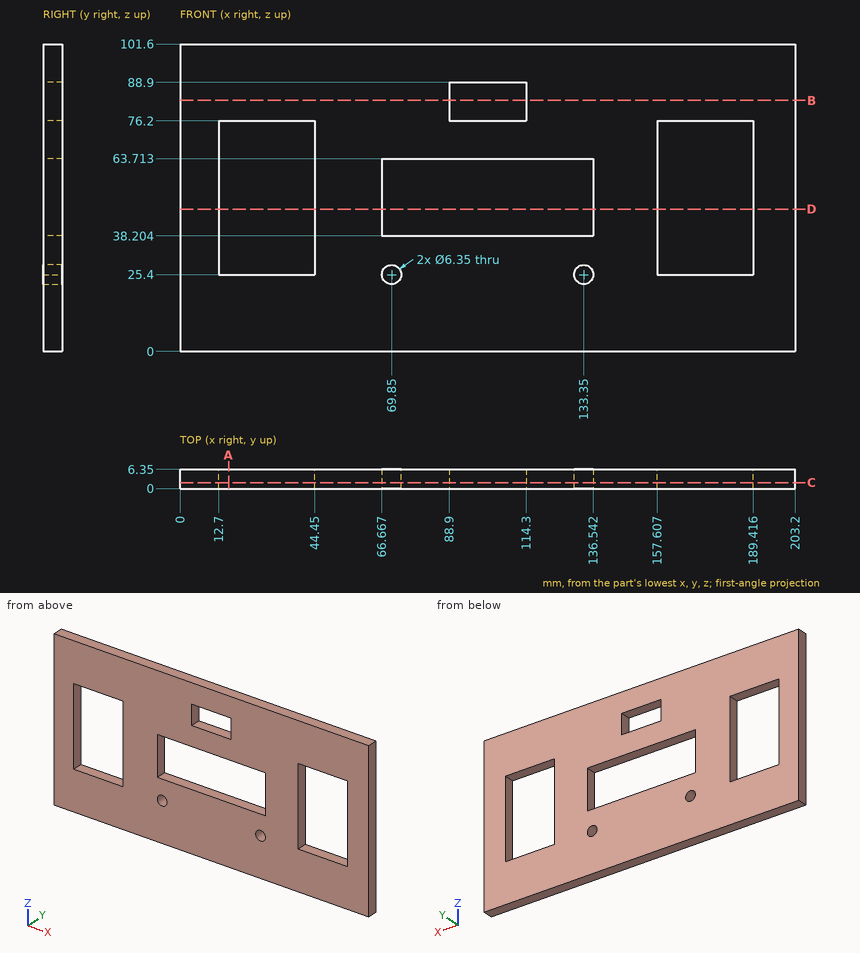
Job drawing, mm, ordinate dimensions from the low corner. One solid piece. Coordinates: 2 decimals unless noted, no trailing zeros. Order: outer loops, then holes, each group sorted by start corner. A loop starts at its lowest first (then second) coordinate and runs counter-clockwise, first axis right, second up. Notation, with made-up numbers: (60, 78.5) -> (97, 78.5) arc R25 cw to (97, 107.5) -> close; hole circle Ø10 at (43.5, -13). An arc over 180 degrees is marked (long way). Put each result on its own line as item: value. Start each with the question number.
(1) Band-saw the part on A-A (x = 16). Give the cut face in (y, z).
(2) Band-saw the part on D-D (z = 47). Give the cut face in (x, y), then the cut area to 3 significant figures.
(3) Probe line 1 along X through (y, z) = (2.75, 51.5); line 2 along Z through (x, y) = (109, 4) (1 decimal); line 3 along X through (y, z) = (1, 76). List the from-to ranges inside material, lowest first. Write a range as [from, to].
(4) Band-saw the part on B-B (z = 83). Give the cut face in (x, y).
(5) Band-saw the part on C-C (y = 2). Count the separate pieces of the cut face and the enclosed holes in it, then the cut area to 3 significant figures.
Determined:
1. outline: (0, 0) -> (6.35, 0) -> (6.35, 25.4) -> (0, 25.4) -> close; (0, 76.2) -> (6.35, 76.2) -> (6.35, 101.6) -> (0, 101.6) -> close
2. outline: (0, 0) -> (12.7, 0) -> (12.7, 6.35) -> (0, 6.35) -> close; (44.45, 0) -> (66.67, 0) -> (66.67, 6.35) -> (44.45, 6.35) -> close; (136.54, 0) -> (157.61, 0) -> (157.61, 6.35) -> (136.54, 6.35) -> close; (189.42, 0) -> (203.2, 0) -> (203.2, 6.35) -> (189.42, 6.35) -> close
2. area: 443 mm²
3. line 1: x = [0, 12.7], [44.45, 66.67], [136.54, 157.61], [189.42, 203.2]
3. line 2: z = [0, 38.2], [63.7, 76.2], [88.9, 101.6]
3. line 3: x = [0, 12.7], [44.45, 157.61], [189.42, 203.2]
4. outline: (0, 0) -> (88.9, 0) -> (88.9, 6.35) -> (0, 6.35) -> close; (114.3, 0) -> (203.2, 0) -> (203.2, 6.35) -> (114.3, 6.35) -> close
5. separate pieces: 1
5. enclosed holes: 6
5. area: 15,200 mm²
